Read the model definition and answer for the solid it produces. Units are mm, in the model's axes. A direction names the side the tool comes from. Coordinates: 2 decimals unless noted, no trailing zeros. Order: outer loops, then holes, each group sorted by start corner. A loop starts at its lowest first (then second) coordinate and runs counter-clockwise, first axis right, second up. Notation, with made-up numbers: M 12,78 L 46,78 A31 ccw 46,102 Z; hole C 24,89 d11. An arc over 180 degrees is marked long. One line per question, with ' | ' between items. Start each with the question number.
1) Find section D-D, the plane x = 2. Count the separate pieces of the cut face and the enclosed holes in it, plus the area to 3 significant figures.
2) Given P1, Ø3, axis at x = 4.5, y = 68.5, coming from the -Z side, flat-ended and moving along its own axis, determine where the tip first touches the part or whether it passes through.
3) A tool of negligible diameter and unlimited length cuts with its end or side. For faces 4 (the face through (3, 257.175, 190)), 5 (the face through (3, 120, 153.988)), from which of +Z, -Z, +X, -X, +Y, -Y can it reach the whole face along a straight path? Write none if from no direction.
4) The mould has two halves that part along Z. Classify faces 1 (the face through (3.131, 163.588, 167.19)), 2 (the face through (3, 129, 279.4)), 3 (the face through (3, -3.175, 138)): +Z half, -Z half, draft (parallel to the pull), parting line (faces both ways), or undercut.
5) Find section B-B, the plane z = 199.5. Write down the section's boundary in (x, y) (3 decimals).
6) Find section C-C, the plane z = 19.05. Write down the section's boundary in (x, y) (3 decimals).
7) Consider probe 1 along Y at (x, z) = (4, 239.5) (3 decimals); probe 2 along Y at (x, z) = (1.5, 203.2) (3 decimals); probe 3 along Y at (x, z) = (1, 187.5) (3 decimals). Determine where each line is inside the solid, lowest interval first.
8) Find section A-A, the plane y = 241.3. Write down the section's boundary in (x, z).
from build123d import *

# Parameters (mm, degrees)
BOSS_EXTRUDE1_DEPTH     = 6.35
F_1_4_CLEARANCE_HOLE4_D = 6.7564
F_1_4_CLEARANCE_HOLE5_D = 6.7564
FILLET4_R               = 101.6
SKETCH22_W              = 63.5
SKETCH22_H              = 69.85
SKETCH22_H_2            = 31.75
CUT_EXTRUDE1_DEPTH      = 7.35
F_5_8_CLEARANCE_HOLE1_D = 16.66748
FILLET5_R               = 6.35
FILLET6_R               = 4.7625


with BuildPart() as part:
    # Sketch1 → Boss-Extrude1 (new body)
    with BuildSketch(Plane(origin=(0, 0, 0), x_dir=(0, 0, -1), z_dir=(1, 0, 0))):
        Polygon((-279.4, 0), (-279.4, 257.175), (-101.6, 257.175), (0, 76.2), (0, 0), (0, -3.175), (-279.4, -3.175), align=None)
    extrude(amount=BOSS_EXTRUDE1_DEPTH)

    # 1/4 Clearance Hole4 (through all)
    with Locations(Plane(origin=(6.35, 0, 0), x_dir=(0, 0, -1), z_dir=(1, 0, 0))):
        with Locations((-266.7, 241.3), (-114.3, 241.3)):
            Hole(F_1_4_CLEARANCE_HOLE4_D / 2)

    # 1/4 Clearance Hole5 (through all)
    with Locations(Plane.ZY):
        with Locations((19.05, 19.05), (260.35, 19.05)):
            Hole(F_1_4_CLEARANCE_HOLE5_D / 2)

    # Fillet4
    fillet4_edges = [part.edges().sort_by_distance(p)[0] for p in [
        (3.175, 76.2, 0),
    ]]
    fillet(fillet4_edges, radius=FILLET4_R)

    # Sketch22 → Cut-Extrude1 (cut, through all)
    with BuildSketch(Plane(origin=(6.35, 0, 0), x_dir=(0, 0, -1), z_dir=(1, 0, 0))):
        with Locations((-185.7375, 50.8)):
            Rectangle(SKETCH22_W, SKETCH22_H)
        with Locations((-185.7375, 120.65)):
            Rectangle(SKETCH22_W, SKETCH22_H_2)
    extrude(amount=-CUT_EXTRUDE1_DEPTH, mode=Mode.SUBTRACT)

    # 5/8 Clearance Hole1 (through all)
    with Locations(Plane(origin=(6.35, 0, 0), x_dir=(0, 0, -1), z_dir=(1, 0, 0))):
        with Locations((-239.7125, 228.6), (-131.7625, 228.6), (-239.7125, 25.4), (-131.7625, 25.4), (-203.2, 155.324999992), (-168.275, 155.324999992)):
            Hole(F_5_8_CLEARANCE_HOLE1_D / 2)

    # Fillet5
    fillet5_edges = [part.edges().sort_by_distance(p)[0] for p in [
        (3.175, -3.175, 0),
        (3.175, -3.175, 279.4),
        (3.175, 257.175, 279.4),
        (3.175, 257.175, 101.6),
    ]]
    fillet(fillet5_edges, radius=FILLET5_R)

    # Fillet6
    fillet6_edges = [part.edges().sort_by_distance(p)[0] for p in [
        (3.175, 15.875, 217.4875),
        (3.175, 85.725, 217.4875),
        (3.175, 85.725, 153.9875),
        (3.175, 15.875, 153.9875),
        (3.175, 104.775, 217.4875),
        (3.175, 136.525, 217.4875),
        (3.175, 136.525, 153.9875),
        (3.175, 104.775, 153.9875),
    ]]
    fillet(fillet6_edges, radius=FILLET6_R)


solid = part.part
Report:
1) separate pieces: 1 | enclosed holes: 12 | area: 55,600 mm^2
2) P1: stops at z = 1.5
3) face 4: +Z, -Z, +X, -X, +Y | face 5: +X, -X
4) face 1: undercut | face 2: +Z half | face 3: draft
5) outline: M 0,-3.175 L 6.35,-3.175 L 6.35,15.875 L 0,15.875 Z; M 0,85.725 L 6.35,85.725 L 6.35,104.775 L 0,104.775 Z; M 0,136.525 L 6.35,136.525 L 6.35,147.858 L 0,147.858 Z; M 0,162.792 L 6.35,162.792 L 6.35,257.175 L 0,257.175 Z
6) outline: M 0,-3.175 L 6.35,-3.175 L 6.35,15.672 L 0,15.672 Z; M 0,22.428 L 6.35,22.428 L 6.35,110.133 L 0,110.133 Z
7) probe 1: y = -3.175 to 17.069, 33.731 to 220.269, 236.931 to 257.175 | probe 2: y = -3.175 to 15.875, 85.725 to 104.775, 136.525 to 146.991, 163.659 to 257.175 | probe 3: y = -3.175 to 15.875, 85.725 to 104.775, 136.525 to 257.175
8) outline: M 0,92.69 L 6.35,92.69 L 6.35,110.92 L 0,110.92 Z; M 0,117.68 L 6.35,117.68 L 6.35,263.32 L 0,263.32 Z; M 0,270.08 L 6.35,270.08 L 6.35,279.4 L 0,279.4 Z
